For this review, take the finished solid that the model builds, in its own axes (mm). A direction names the side the tool comes from. Coordinates: 2 decimals unless noted, no trailing zeros. Order: outer loops, then holes, each group sorted by start corner. A loop starts at its lowest first (then second) coordinate and runs counter-clockwise, first axis right, second up. Notation, with made-up numbers: (65.5, 79.5) - (82.5, 79.5) arc R25 cw to (82.5, 118.5) - close; hole circle Ø9 at (71.5, 62). An arc over 180 degrees is marked (long way). One line per item, written item: value. Start each with the question number.
(1) Clearance check with flat-ended pins moving along their axes: pin 1 (1 mm diameter, centred on y = 1.5, z = 5.5, fed in from +X); pin 2 (4 mm diameter, centred on y = 2.5, z = 4.5, fed in from -X); pin 3 (3 mm diameter, centred on y = 2, z = 27, fed in from +X). State where each tip first meets the part, or that it passes through.
(2) Consider section A-A on z = 24. Write out the cut boundary in (x, y).
(3) For faces 1 (the flat face through (-1, -1, -2.21)), 2 (the flat face through (0, 1.191, -1)), list the 3-axis set-ups (+Z, -Z, +X, -X, +Y, -Y) from which the entire face can be reached by the end or side of a thin tool; tool diameter is ignored.
(4) To check wall thickness, follow line 1 along Y through (x, z) = (-0.5, 38.5); line 2 along Z through (x, y) = (-0.5, 0.25). State the ranges of each line that lie inside material, in increasing order.
(5) Mouldability with a two-part tool opening along Y and no side actions: class faces 3 (the cylindrical face through (1.987, -0.626, 24.794)), 4 (the flat face through (1.036, 0.587, -1.427)), 5 (the flat face through (-2, -2, 0)) as released by +Y, released by -Y, zero draft, split by the parting line, or undercut.
Autodesk Inventor part; units mm, degrees
ref_plane "YZ Plane" through (0, 0, 0) normal (1, 0, 0) x (0, 1, 0)
ref_plane "XZ Plane" through (0, 0, 0) normal (0, 1, 0) x (-1, 0, 0)
ref_plane "XY Plane" through (0, 0, 0) normal (0, 0, 1) x (1, 0, 0)
sketch "Sketch1" plane through (0, 0, 0) normal (0, 0, 1) x (1, 0, 0)
  circle A0 centre (0, 0) radius 2.0828
  dimension "d0" = 4.1656
extrude "Extrusion1" add sketch "Sketch1" along normal blind 50.8
sketch "Sketch2" plane through (0, 0, 0) normal (0, 1, 0) x (-1, 0, 0)
  line L0 (0, 0) -> (0, -2.2098)
  line L1 (0, 0) -> (3.9624, 0)
  line L2 (0, -2.2098) -> (2.032, -2.2098)
  line L3 (3.9624, 0) -> (3.9624, 3.6562) construction
  arc A0 (2.032, -2.2098) -> (3.9624, -0.4599) centre (0.1837, 1.7689) ccw
  line L4 (4.5847, 0.6553) -> (4.5847, -0.2608) construction
  line L5 (3.9624, -0.4599) -> (3.9624, 0)
  dimension "d3" = 2.2098
  dimension "d6" = 2.032
  dimension "d19" = 3.9624
revolve "Revolution1" add sketch "Sketch2" angle 360 about axis through (0, 0, 0) along (0, 0, -1)
sketch "Sketch3" plane through (0, 0, -2.2098) normal (0, 0, -1) x (-1, 0, 0)
  circle A0 centre (0, 0) radius 2.032
  line L0 (-0.6874, 1.1906) -> (0.6874, 1.1906)
  line L1 (0.6874, 1.1906) -> (1.3748, 0)
  line L2 (1.3748, 0) -> (0.6874, -1.1906)
  line L3 (0.6874, -1.1906) -> (-0.6874, -1.1906)
  line L4 (-0.6874, -1.1906) -> (-1.3748, 0)
  line L5 (-1.3748, 0) -> (-0.6874, 1.1906)
  dimension "d8" = 2.3813
extrude "Extrusion2" cut sketch "Sketch3" against normal blind 1.5875 contours L0 L1 L2 L3 L4 L5
chamfer "Chamfer1" distance 0.508 angle 45 1 edges at (-2.0828, 0, 50.8)
thread "Thread1"
properties part number "10-32 x500 button head" material "Aluminum 6061"
Geometry check:
1. pin 1: stops at x = 1.83
1. pin 2: stops at x = -2.02
1. pin 3: stops at x = 2.02
2. outline: circle Ø4.17 at (0, 0)
3. face 1: -Z, +X, -X, +Y, -Y
3. face 2: -Z
4. line 1: y = -2.02 to 2.02
4. line 2: z = -0.62 to 50.8
5. face 3: split by the parting line
5. face 4: undercut
5. face 5: zero draft
